from build123d import *

# Parameters (mm, degrees)
F0_R     = 17.78
F1_DEPTH = 38.1
F2_R     = 15.24
F3_DEPTH = 114.3
F4_R     = 15.24
F5_DEPTH = 31.75
F6_R     = 12.7
F7_DEPTH = 127
F8_SIZE2 = 5.07999
F8_SIZE  = 2.53999


# Not quite as in the source:
# - a fillet or chamfer is up to 0.001 mm smaller than in the source, because OpenCascade refuses the exact size


with BuildPart() as f1:
    # F0 (on Top) → F1 (new body)
    with BuildSketch(Plane.XY):
        Circle(F0_R)
    extrude(amount=F1_DEPTH)

    # F2 (on face) → F3 (join)
    with BuildSketch(Plane.XY.offset(38.1)):
        Circle(F2_R)
    extrude(amount=F3_DEPTH)

    # F4 (on face) → F5 (cut)
    with BuildSketch(Plane(origin=(0, 0, 0), x_dir=(1, 0, 0), z_dir=(0, 0, -1))):
        Circle(F4_R)
    extrude(amount=-F5_DEPTH, mode=Mode.SUBTRACT)

    # F6 (on face) → F7 (cut)
    with BuildSketch(Plane.XY.offset(152.4)):
        Circle(F6_R)
    extrude(amount=-F7_DEPTH, mode=Mode.SUBTRACT)

    # F8 (size 2.54 and 5.08 in the source; OpenCascade refuses exactly that, so slightly less here)
    f8_edges = [f1.edges().sort_by_distance(p)[0] for p in [
        (-17.78, 0, 38.1),
    ]]
    f8_side = f1.faces().sort_by_distance((-17.277106, 0, 38.1))[0]
    chamfer(f8_edges, length=F8_SIZE, length2=F8_SIZE2, reference=f8_side)


solid = f1.part
Here's how the part is built. I have some questions about the finished solid (model axes, mm). A direction names the side the tool comes from. Give positions to 0.01 mm unless a question says otherwise; leave off trailing zeros. Loops run counter-clockwise (first coordinate to the right, second up) from the corner with the lowest first, then second, coordinate; pieces in that order, holes last. Notation, with made-up numbers: (51.5, -26.5) -> (83.5, -26.5) arc R22 cw to (83.5, -20.5) -> close; hole circle Ø3 at (-11, 53). An arc over 180 degrees is marked (long way). Answer as a JSON object with one key per item and string values. Group by question number.
Item 1: I need wall thicknesses on L1, parallel to Y at x = 0, z = 11; L2, parallel to Y at x = 0, z = 113; L3, parallel to Z at x = 0, y = -13. Which ranges of each line are inside material? Lowest first, please.
Item 2: Will these pins go through, and if not, where does the flat tip stop? pin 1 (4 mm diameter, centred on y = 0, z = 130.5, fed in from -X); pin 2 (5 mm diameter, centred on x = -10.5, y = 0, fed in from -Z); pin 3 (8 mm diameter, centred on y = 6.5, z = 95.5, fed in from -X).
Item 3: Imagine slicing it at D-D on z = 10. Write out the boundary of the cut face in (x, y).
Item 4: On a 3-axis mill with a long thin cutter (end or side, diameter ignored), from which of +Z, -Z, +X, -X, +Y, -Y can I reach the whole of each face in a straight line? I mean faces 1 (the flat face through (-3.5, -12.5, 31.75)), 2 (the cylindrical face through (-2.75, -12.4, 92.92)), 3 (the cylindrical face through (-3.3, -14.88, 94.45)). Say none if no direction works.
Item 5: Imagine slicing it at C-C on z = 134. Write out the boundary of the cut face in (x, y), then the cut area to 3 significant figures.
Answer list:
{
 "1": {"L1": "y = -17.78 to -15.24, 15.24 to 17.78", "L2": "y = -15.24 to -12.7, 12.7 to 15.24", "L3": "z = 31.75 to 152.4"},
 "2": {"pin 1": "stops at x = -15.24", "pin 2": "stops at z = 31.75", "pin 3": "stops at x = -15.03"},
 "3": {"outline": "circle Ø35.56 at (0, 0); hole circle Ø30.48 at (0, 0)"},
 "4": {"face 1": "-Z", "face 2": "+Z, -Z", "face 3": "+Z"},
 "5": {"outline": "circle Ø30.48 at (0, 0); hole circle Ø25.4 at (0, 0)", "area": "223 mm2"}
}
